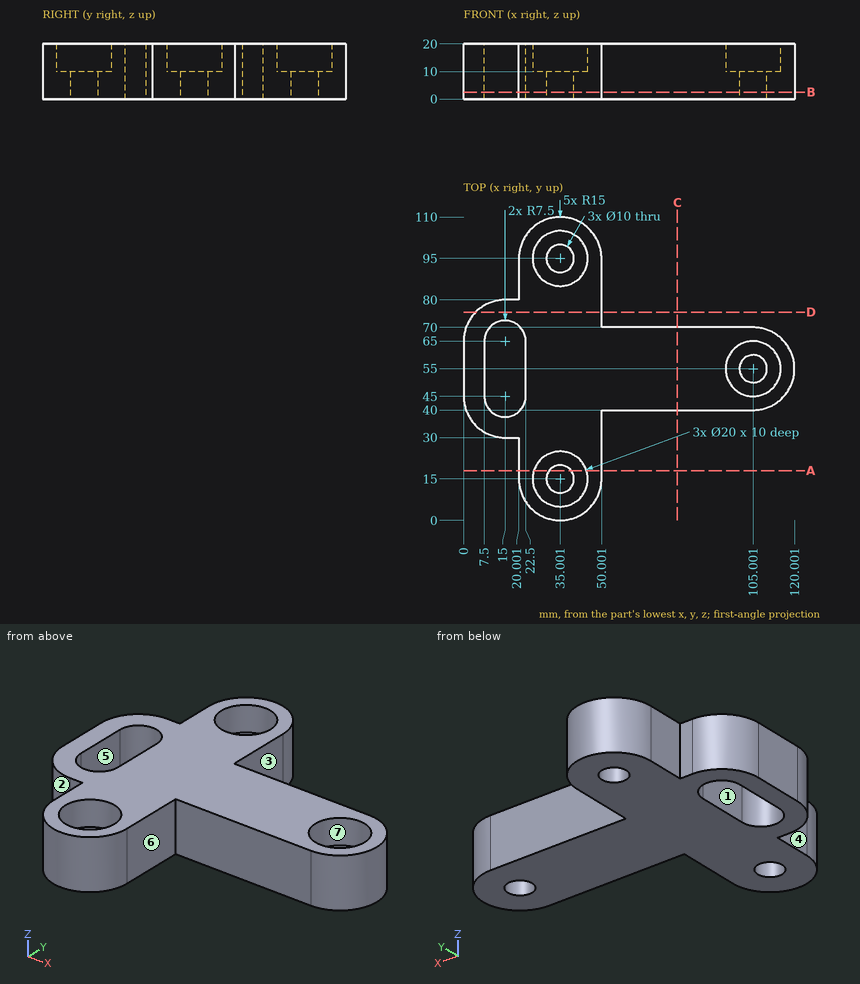
Here's the drawing with two shaded views (mm, measured from the low corner). I have some questions. A direction names the side the tool comes from. Coordinates: 2 decimals unless noted, no trailing zeros. Loops run counter-clockwise (first coordinate to the right, second up) from the corner with the lowest first, then second, coordinate; pieces in that order, holes last. Notation, with made-up numbers: (37.25, 24.5) -> (58.25, 24.5) arc R9 ccw to (58.25, 33.5) -> close; hole circle Ø10 at (52.25, 53.5). An arc over 180 degrees is marked (long way). Use one line per item in the form item = value. Start each with the question number.
(1) If we section it at D-D (y = 75.5): Please give me the cut outline in (x, z), then the cut area to 3 significant figures.
(2) Will these pins go through, and if not, where does the flat tip stop? pin 1 (18 mm diameter, centred on x = 35, y = 95, fed in from -Z); pin 2 (1.5 mm diameter, centred on y = 86, z = 12.5, fed in from +X); pin 3 (2 mm diameter, centred on y = 94, z = 12, fed in from -X); pin 4 (18 mm diameter, centred on x = 105, y = 55, fed in from +Z).
(3) If we section it at C-C (x = 77.5): Please give me the cut outline in (y, z), then the cut area to 3 significant figures.
(4) On a 3-axis mill with a long thin cutter (end or side, diameter ignored), from which of +Z, -Z, +X, -X, +Y, -Y can I reach the whole of each face in a straight line? I mean the marked faces 4, 5, 6 and 7. Say none if no direction works.
(5) If we section it at A-A (y = 18): Please give me the cut outline in (x, z), then the cut area to 3 significant figures.
(6) Please list where these lines run through material, in increasing order: line 1 along Y through (x, z) = (21.5, 10.5) (1 decimal); line 2 along Y through (x, z) = (36, 9); line 3 along X through (y, z) = (83.5, 18).
(7) If we section it at B-B (z = 2.5): Please give me the cut outline in (x, y).
(8) We'd pull the mould along Y, two halves only. Please class the marked faces 1, 2 and 3: pulls with the +Y half, pulls with the -Y half, needs draft (parallel to the pull), parting line crosses it, or undercut.
Verdict:
q1.outline = (4.29, 0) -> (50, 0) -> (50, 20) -> (4.29, 20) -> close
q1.area = 914 mm²
q2.pin_1 = 0
q2.pin_2 = 50
q2.pin_3 = 20
q2.pin_4 = 10
q3.outline = (40, 0) -> (70, 0) -> (70, 20) -> (40, 20) -> close
q3.area = 600 mm²
q4.face_4 = +Z, -Z, -X, -Y
q4.face_5 = +Z, -Z
q4.face_6 = +Z, -Z, +X, -Y
q4.face_7 = +Z
q5.outline = (20, 0) -> (31, 0) -> (31, 10) -> (25.46, 10) -> (25.46, 20) -> (20, 20) -> close; (39, 0) -> (50, 0) -> (50, 20) -> (44.54, 20) -> (44.54, 10) -> (39, 10) -> close
q5.area = 329 mm²
q6.line_1 = 8.5 to 41.3, 68.7 to 101.5
q6.line_2 = 0.03 to 10.1, 19.9 to 90.1, 99.9 to 109.97
q6.line_3 = 20 to 50
q7.outline = (0, 45) arc R15 ccw to (15, 30) -> (20, 30) -> (20, 15) arc R15 ccw to (50, 15) -> (50, 40) -> (105, 40) arc R15 ccw to (105, 70) -> (50, 70) -> (50, 95) arc R15 ccw to (20, 95) -> (20, 80) -> (15, 80) arc R15 ccw to (0, 65) -> close; hole (7.5, 45) arc R7.5 ccw to (22.5, 45) -> (22.5, 65) arc R7.5 ccw to (7.5, 65) -> close; hole circle Ø10 at (35, 15); hole circle Ø10 at (35, 95); hole circle Ø10 at (105, 55)
q8.face_1 = undercut
q8.face_2 = pulls with the -Y half
q8.face_3 = needs draft
